from build123d import *

# Parameters (mm, degrees)
PAD_DEPTH    = 3.25
SKETCH001_W  = 9
SKETCH001_H  = 20
PAD001_DEPTH = 3
CHAMFER_SIZE = 2


with BuildPart() as part:
    # Sketch → Pad (new body)
    with BuildSketch(Plane.XY):
        Polygon((38.1, 0), (38.1, 8), (38.1, 68), (31.45, 68), (31.45, 8), (24.85, 8), (24.85, 41), (13.25, 41), (13.25, 8), (6.65, 8), (6.65, 68), (0, 68), (0, 8), (0, 0), (14.55, 0), (14.55, -20), (23.55, -20), (23.55, 0), align=None)
    extrude(amount=PAD_DEPTH)

    # Sketch001 (on Face20 of Pad) → Pad001 (join)
    with BuildSketch(Plane.XY.offset(3.25)):
        with Locations((19.05, -10)):
            Rectangle(SKETCH001_W, SKETCH001_H)
    extrude(amount=PAD001_DEPTH)

    # Chamfer
    chamfer_edges = [part.edges().sort_by_distance(p)[0] for p in [
        (19.05, -20, 6.25),
    ]]
    chamfer(chamfer_edges, length=CHAMFER_SIZE)


solid = part.part
Geometry: final body of the model. Coordinates: model frame, mm. A direction names the side the tool comes from. Give positions to 0.01 mm unless a question says otherwise; leave off trailing zeros. Order: outer loops, then holes, each group sorted by start corner. A loop starts at its lowest first (then second) coordinate and runs counter-clockwise, first axis right, second up. Notation, with made-up numbers: (59.25, -5) -> (98.25, -5) arc R13 cw to (98.25, 1) -> close; hole circle Ø7 at (74, 60.25). An arc over 180 degrees is marked (long way). Answer as a JSON object with one key per item and string values.
Q1. Section C-C (z = 1.5). Output: boundary loops of the cut face in (x, y), plus the area to 3 significant figures.
Entries:
{"outline": "(0, 0) -> (14.55, 0) -> (14.55, -20) -> (23.55, -20) -> (23.55, 0) -> (38.1, 0) -> (38.1, 68) -> (31.45, 68) -> (31.45, 8) -> (24.85, 8) -> (24.85, 41) -> (13.25, 41) -> (13.25, 8) -> (6.65, 8) -> (6.65, 68) -> (0, 68) -> close", "area": "1,670 mm^2"}
Q2. Access query for faces 1 (the flat face through (24.85, 24, 2)), 2 (the flat face through (19, 27, 3.25)), 3 (the flat face through (7, 0, 2)). Directions: +Z, -Z, +X, -X, +Y, -Y. A direction counts if a zero-diameter tool reaches every point of the face in a straight line with its end or side. Return the directions, or none.
Entries:
{"face 1": "+Z, -Z, +Y", "face 2": "+Z, +X, -X, +Y", "face 3": "+Z, -Z, -X, -Y"}
Q3. Section D-D (x = 19). Output: boundary loops of the cut face in (y, z).
Entries:
{"outline": "(-20, 0) -> (41, 0) -> (41, 3.25) -> (0, 3.25) -> (0, 6.25) -> (-18, 6.25) -> (-20, 4.25) -> close"}
Q4. Section A-A (y = 23). Output: boundary loops of the cut face in (x, z), plus the area to 3 significant figures.
Entries:
{"outline": "(0, 0) -> (6.65, 0) -> (6.65, 3.25) -> (0, 3.25) -> close; (13.25, 0) -> (24.85, 0) -> (24.85, 3.25) -> (13.25, 3.25) -> close; (31.45, 0) -> (38.1, 0) -> (38.1, 3.25) -> (31.45, 3.25) -> close", "area": "80.9 mm^2"}
Q5. Material intervals for probe 1 along X at (y, z) = (43, 2); probe 2 along Z at (x, y) = (35.5, 45); probe 3 along Y at (x, z) = (31, 1.75), sorted ascending.
Entries:
{"probe 1": "x = 0 to 6.65, 31.45 to 38.1", "probe 2": "z = 0 to 3.25", "probe 3": "y = 0 to 8"}
Q6. First-contact query: pin 1 (2.5 mm diameter, centred on x = 21.5, z = 2, fed in from +Y); pin 2 (3.5 mm diameter, centred on x = 34, z = 1.5, fed in from -Y); pin 3 (0.9 mm diameter, centred on x = 19, z = 5, fed in from +Y). Flat tips, straight axial feed; report the tip coordinate or a pass-through.
Entries:
{"pin 1": "stops at y = 41", "pin 2": "stops at y = 0", "pin 3": "stops at y = 0"}
Q7. Section B-B (y = 46). Output: boundary loops of the cut face in (x, z).
Entries:
{"outline": "(0, 0) -> (6.65, 0) -> (6.65, 3.25) -> (0, 3.25) -> close; (31.45, 0) -> (38.1, 0) -> (38.1, 3.25) -> (31.45, 3.25) -> close"}
